Source: CAD feature listing. Evaluate the final solid. Frame: model axes, mm. Face numbers are marked on the shaded views. A direction names the side the tool comes from. Round coordinates to 2 decimals unless told otherwise and drop trailing zeros. Write each loop counter-clockwise with the first axis right and the second up, starting at its lowest first coordinate (ties: lowest second). Pieces come first, ordered by that corner, then holes. Notation, with made-up numbers: (81.25, -11) -> (95.25, -11) arc R18 ccw to (95.25, 14) -> close; hole circle Ø3 at (76, 57). An arc over 180 degrees is marked (long way). Return JSON: item names as keys, results as strings. Group by question number.
from build123d import *

# Parameters (mm, degrees)
SKETCH_1_W          = 40
SKETCH_1_H          = 20
SKETCH_1_W_2        = 36
SKETCH_1_H_2        = 16
EXTRUDE_1_DEPTH     = 50
SKETCH_2_R          = 7
CUT_EXTRUDE_1_DEPTH = 20
SKETCH_3_R          = 1.5
CUT_EXTRUDE_2_DEPTH = 50


with BuildPart() as part:
    # 草图1 → 凸台-拉伸1 (new body)
    with BuildSketch(Plane.XY):
        Rectangle(SKETCH_1_W, SKETCH_1_H)
        Rectangle(SKETCH_1_W_2, SKETCH_1_H_2, mode=Mode.SUBTRACT)
    extrude(amount=EXTRUDE_1_DEPTH)

    # 草图2 → 切除-拉伸1 (cut)
    with BuildSketch(Plane(origin=(0, 10, 0), x_dir=(1, 0, 0), z_dir=(0, 1, 0))):
        with Locations(Location((5, -20, 0), (0, 0, 270))):
            Circle(SKETCH_2_R)
    extrude(amount=-CUT_EXTRUDE_1_DEPTH, mode=Mode.SUBTRACT)

    # 草图3 → 切除-拉伸2 (cut)
    with BuildSketch(Plane(origin=(20, 0, 0), x_dir=(0, 0, -1), z_dir=(1, 0, 0))):
        with Locations(Location((-6, 0, 0), (0, 0, 90))):
            Circle(SKETCH_3_R)
        with Locations(Location((-33, 0, 0), (0, 0, 90))):
            Circle(SKETCH_3_R)
        with Locations(Location((-45, 0, 0), (0, 0, 90))):
            Circle(SKETCH_3_R)
    extrude(amount=-CUT_EXTRUDE_2_DEPTH, mode=Mode.SUBTRACT)


solid = part.part
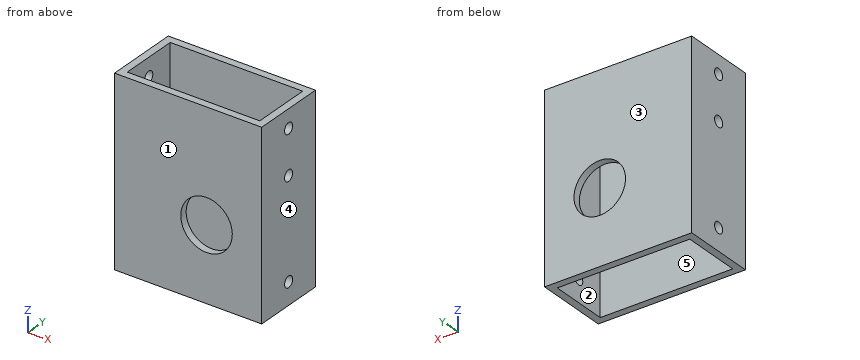
Item 1: Cut plane C-C on x = -3. Output: boundary loops of the cut face in (y, z).
Item 2: Cut plane B-B on z = 6. Output: boundary loops of the cut face in (x, y), and give its area (3 significant figures).
Item 3: Material intervals for probe 1 along Z at (x, y) = (18.5, 0); probe 2 along X at (y, z) = (2.5, 26); probe 3 along Y at (x, z) = (-14.5, 10.5), sorted ascending.
Item 4: Cut plane D-D on x = 5. Output: boundary loops of the cut face in (y, z), and give its area (3 significant figures).
Item 5: Set-up query: the marked faces 4 and 5. Return all of +Z, -Z, +X, -X, +Y, -Y with unobstructed straight access to the full face (end or side cutting, diameter ignored); none if empty.
Item 6: Cut plane A-A on y = 0. Give the number of separate pieces and of enclosed holes in the cut face, and give its area (3 significant figures).
Item 7: Pull-direction query (Y, two-part tool) for the marked faces 1, 2 and 3; classes: +Y half, -Y half, draft (parallel to the pull), parting line (faces both ways), or undercut.
Here are the results:
{
 "1": {"outline": "(-10, 0) -> (-8, 0) -> (-8, 50) -> (-10, 50) -> close; (8, 0) -> (10, 0) -> (10, 50) -> (8, 50) -> close"},
 "2": {"outline": "(-20, -10) -> (20, -10) -> (20, -1.5) -> (18, -1.5) -> (18, -8) -> (-18, -8) -> (-18, -1.5) -> (-20, -1.5) -> close; (-20, 1.5) -> (-18, 1.5) -> (-18, 8) -> (18, 8) -> (18, 1.5) -> (20, 1.5) -> (20, 10) -> (-20, 10) -> close", "area": "212 mm^2"},
 "3": {"probe 1": "z = 0 to 4.5, 7.5 to 31.5, 34.5 to 43.5, 46.5 to 50", "probe 2": "x = -20 to -18, 18 to 20", "probe 3": "y = -10 to -8, 8 to 10"},
 "4": {"outline": "(-10, 0) -> (-8, 0) -> (-8, 13) -> (-10, 13) -> close; (-10, 27) -> (-8, 27) -> (-8, 50) -> (-10, 50) -> close; (8, 0) -> (10, 0) -> (10, 13) -> (8, 13) -> close; (8, 27) -> (10, 27) -> (10, 50) -> (8, 50) -> close", "area": "144 mm^2"},
 "5": {"face 4": "+Z, -Z, +X, +Y, -Y", "face 5": "+Z, -Z"},
 "6": {"separate pieces": "8", "enclosed holes": "0", "area": "164 mm^2"},
 "7": {"face 1": "-Y half", "face 2": "undercut", "face 3": "+Y half"}
}
